CAD build for the part. Positions are in the model's coordinates, mm. Give positions to 0.01 mm unless a question says otherwise; leave off trailing zeros. Loops run counter-clockwise (first coordinate to the right, second up) from the corner with the lowest first, then second, coordinate; pieces in that order, holes last. Notation, with made-up numbers: M -23,38.5 L -10,38.5 A19 cw -10,75.5 Z; hole C 81.25,7.25 d4. An arc over 180 degrees is marked long. One line per question, with ' | ' between items.
```python
from build123d import *

# Parameters (mm, degrees)
SZKIC1_R                    = 3
SZKIC1_R_2                  = 3.25
SZKIC1_R_3                  = 2.5
DODANIE_WYCI_GNI_CIE1_DEPTH = 10
ZAOKR_GLENIE1_R             = 4100


with BuildPart() as part:
    # Szkic1 → Dodanie-wyciągnięcie1 (new body)
    with BuildSketch(Plane(origin=(0, 0, 0), x_dir=(1, 0, 0), z_dir=(0, 1, 0))):
        Polygon((200, 0), (200, 20), (100, 20), (0, 24), (0, -4), (100, 0), align=None)
        with Locations(Location((100, 10, 0), (0, 0, 270))):
            Circle(SZKIC1_R, mode=Mode.SUBTRACT)
        with Locations(Location((190, 10, 0), (0, 0, 270))):
            Circle(SZKIC1_R_2, mode=Mode.SUBTRACT)
        with Locations(Location((10, 17, 0), (0, 0, 270))):
            Circle(SZKIC1_R_3, mode=Mode.SUBTRACT)
        with Locations(Location((10, 3, 0), (0, 0, 270))):
            Circle(SZKIC1_R_3, mode=Mode.SUBTRACT)
        with BuildLine():
            Line((22.984822323, 15.57457628), (86.25939238, 15.57457628))
            ThreePointArc((86.25939238, 15.57457628), (89.794926286, 14.110110186), (91.25939238, 10.57457628))
            Line((91.25939238, 10.57457628), (91.25939238, 9.696719379))
            ThreePointArc((91.25939238, 9.696719379), (89.794926286, 6.161185473), (86.25939238, 4.696719379))
            Line((86.25939238, 4.696719379), (22.984822323, 4.696719379))
            ThreePointArc((22.984822323, 4.696719379), (19.449288417, 6.161185473), (17.984822323, 9.696719379))
            Line((17.984822323, 9.696719379), (17.984822323, 10.57457628))
            ThreePointArc((17.984822323, 10.57457628), (19.449288417, 14.110110186), (22.984822323, 15.57457628))
        make_face(mode=Mode.SUBTRACT)
        with BuildLine():
            Line((113.225148066, 15.57457628), (176.286209663, 15.57457628))
            ThreePointArc((176.286209663, 15.57457628), (179.821743569, 14.110110186), (181.286209663, 10.57457628))
            Line((181.286209663, 10.57457628), (181.286209663, 9.752776346))
            ThreePointArc((181.286209663, 9.752776346), (179.821743569, 6.21724244), (176.286209663, 4.752776346))
            Line((176.286209663, 4.752776346), (113.225148066, 4.752776346))
            ThreePointArc((113.225148066, 4.752776346), (109.68961416, 6.21724244), (108.225148066, 9.752776346))
            Line((108.225148066, 9.752776346), (108.225148066, 10.57457628))
            ThreePointArc((108.225148066, 10.57457628), (109.68961416, 14.110110186), (113.225148066, 15.57457628))
        make_face(mode=Mode.SUBTRACT)
    extrude(amount=DODANIE_WYCI_GNI_CIE1_DEPTH)

    # Zaokrąglenie1
    # the kernel refuses this fillet: 4100 mm, written as the material it adds along each edge
    with BuildSketch(Plane(origin=(100, 0, -20), x_dir=(1, 0, 0), z_dir=(0, 1, 0)), Plane(origin=(100, 0, 0), x_dir=(-0.9992009587217893, 0, 0.03996803834887583), z_dir=(0, 1, 0))) as zaokr_glenie1_piece_1:
        with BuildLine():
            CenterArc((ZAOKR_GLENIE1_R * 0.0199920063936, ZAOKR_GLENIE1_R), ZAOKR_GLENIE1_R, 267.709389957, 2.290610043)
            Line((-ZAOKR_GLENIE1_R * 0.0199760319553, ZAOKR_GLENIE1_R * 0.000799041278211), (0, 0))
            Line((0, 0), (ZAOKR_GLENIE1_R * 0.0199920063936, 0))
        make_face()
    extrude(amount=10)


solid = part.part
```
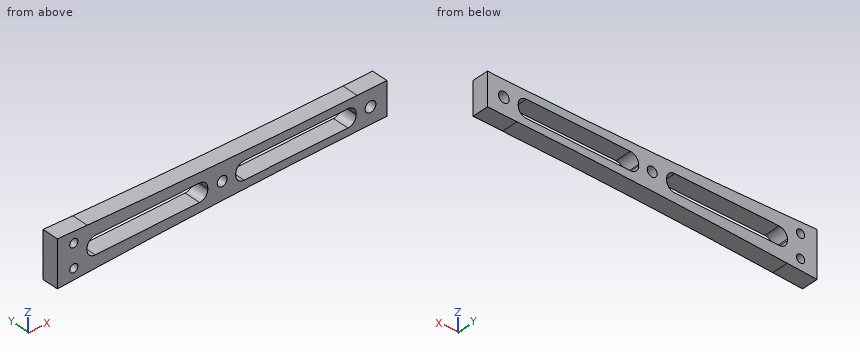
Item 1: Drop flat-ended pins along their axis: P1, Ø3, axis at x = 193, y = 7, coming from the +Z side; P2, Ø1, axis at y = 3, z = -10, coming from the -X side; P3, Ø5, axis at x = 62, y = 5, coming from the -Z side. Give the stop position or say it passes through.
Conclusion:
P1: z = 0 | P2: x = 0 | P3: z = -21.83
Item 2: Saw through at A-A on x = 10. Give the cut face in (y, z), and give its area (3 significant figures).
Conclusion:
outline: M 0,-23.6 L 10,-23.6 L 10,-19.5 L 0,-19.5 Z; M 0,-14.5 L 10,-14.5 L 10,-5.5 L 0,-5.5 Z; M 0,-0.5 L 10,-0.5 L 10,3.6 L 0,3.6 Z | area: 172 mm²
Item 3: Drill centre lines: line 1 along X through (y, z) = (4.25, -10); line 2 along X through (y, z) = (7, -17); line 3 along Z through (x, y) = (11.5, 4.5). Where is each one in solid material? Low to high. Write a range as [from, to].
Conclusion:
line 1: [0, 17.98], [91.26, 97], [103, 108.23], [181.29, 186.75], [193.25, 200] | line 2: [0, 7.5], [12.5, 200] | line 3: [-23.54, -19], [-15, -5], [-1, 3.54]
Item 4: Saw through at D-D on x = 35. Give the cut face in (y, z).
Conclusion:
outline: M 0,-22.63 L 10,-22.63 L 10,-15.57 L 0,-15.57 Z; M 0,-4.7 L 10,-4.7 L 10,2.63 L 0,2.63 Z
Item 5: Saw through at B-B on y = 8.5. Give the cut face in (x, z), and give its area (3 significant figures).
Conclusion:
outline: M 0,-24 L 18.1,-23.28 A4100 cw 181.97,-20 L 200,-20 L 200,0 L 181.97,0 A4100 cw 18.1,3.28 L 0,4 Z; hole C 10,-17 d5; hole C 10,-3 d5; hole M 17.98,-10.57 A5 ccw 22.98,-15.57 L 86.26,-15.57 A5 ccw 91.26,-10.57 L 91.26,-9.7 A5 ccw 86.26,-4.7 L 22.98,-4.7 A5 ccw 17.98,-9.7 Z; hole C 100,-10 d6; hole M 108.23,-10.57 A5 ccw 113.23,-15.57 L 176.29,-15.57 A5 ccw 181.29,-10.57 L 181.29,-9.75 A5 ccw 176.29,-4.75 L 113.23,-4.75 A5 ccw 108.23,-9.75 Z; hole C 190,-10 d6.5 | area: 2,840 mm²
Item 6: Saw through at C-C on x = 58.5. Give the cut face in (y, z).
Conclusion:
outline: M 0,-21.86 L 10,-21.86 L 10,-15.57 L 0,-15.57 Z; M 0,-4.7 L 10,-4.7 L 10,1.86 L 0,1.86 Z
